```python
from build123d import *

# Parameters (mm, degrees)
SKETCH030_R             = 11
PAD011_DEPTH            = 8.5
SKETCH031_R             = 9.85
PAD012_DEPTH            = 2.5
SKETCH032_R             = 9
POCKET019_DEPTH         = 7.5
SKETCH033_R             = 1.95
POCKET020_DEPTH         = 1.5
FILLET010_R             = 1.2
SKETCH034_R             = 1.1
POCKET021_DEPTH         = 2
SKETCH035_R             = 3.3
POCKET022_DEPTH         = 3.5
SKETCH036_R             = 4.1
POCKET023_DEPTH         = 1.4
BODY011_PLACEMENT_ANGLE = 180.00001


with BuildPart() as part:
    # Sketch030 → Pad011 (new body)
    with BuildSketch(Plane.XY):
        Circle(SKETCH030_R)
    extrude(amount=PAD011_DEPTH)

    # Sketch031 (on Face3 of Pad011) → Pad012 (join)
    with BuildSketch(Plane.XY.offset(8.5)):
        Circle(SKETCH031_R)
    extrude(amount=PAD012_DEPTH)

    # Sketch032 (on Face5 of Pad012) → Pocket019 (cut)
    with BuildSketch(Plane.XY.offset(11)):
        Circle(SKETCH032_R)
    extrude(amount=-POCKET019_DEPTH, mode=Mode.SUBTRACT)

    # Sketch033 (on Face2 of Pocket019) → Pocket020 (cut)
    with BuildSketch(Plane(origin=(0, 0, 0), x_dir=(1, 0, 0), z_dir=(0, 0, -1))):
        with Locations((0, 6.8)):
            Circle(SKETCH033_R)
        with Locations((-5.8889727457, -3.4)):
            Circle(SKETCH033_R)
        with Locations((5.8889727457, -3.4)):
            Circle(SKETCH033_R)
    extrude(amount=-POCKET020_DEPTH, mode=Mode.SUBTRACT)

    # Fillet010
    fillet010_edges = [part.edges().sort_by_distance(p)[0] for p in [
        (-11, 0, 0),
    ]]
    fillet(fillet010_edges, radius=FILLET010_R)

    # Sketch034 (on Face11 of Fillet010) → Pocket021 (cut)
    with BuildSketch(Plane(origin=(0, 0, 1.5), x_dir=(1, 0, 0), z_dir=(0, 0, -1))):
        with Locations((-5.8889727457, -3.4)):
            Circle(SKETCH034_R)
        with Locations((0, 6.8)):
            Circle(SKETCH034_R)
        with Locations((5.8889727457, -3.4)):
            Circle(SKETCH034_R)
    extrude(amount=-POCKET021_DEPTH, mode=Mode.SUBTRACT)

    # Sketch035 (on Face4 of Pocket021) → Pocket022 (cut)
    with BuildSketch(Plane(origin=(0, 0, 0), x_dir=(1, 0, 0), z_dir=(0, 0, -1))):
        Circle(SKETCH035_R)
        with BuildLine():
            ThreePointArc((-3.5353318533, 4.2132444372), (-3.3874236532, 5.9038429005), (-5.0780221165, 6.0517511006))
            ThreePointArc((-5.0780221165, 6.0517511006), (-6.8416006899, 3.95), (-7.7799812488, 1.3718206036))
            ThreePointArc((-7.7799812488, 1.3718206036), (-6.8065897584, -0.0183265132), (-5.4164426416, 0.9550649772))
            ThreePointArc((-3.5353318533, 4.2132444372), (-4.7631397208, 2.75), (-5.4164426416, 0.9550649772))
        make_face()
        with BuildLine():
            ThreePointArc((5.0780221165, 6.0517511006), (3.3874236532, 5.9038429005), (3.5353318533, 4.2132444372))
            ThreePointArc((5.4164426416, 0.9550649772), (4.7631397208, 2.75), (3.5353318533, 4.2132444372))
            ThreePointArc((5.4164426416, 0.9550649772), (6.8065897584, -0.0183265132), (7.7799812488, 1.3718206036))
            ThreePointArc((7.7799812488, 1.3718206036), (6.8416006899, 3.95), (5.0780221165, 6.0517511006))
        make_face()
        with BuildLine():
            ThreePointArc((-1.8811107883, -5.1683094143), (-3.4191661052, -5.8855163873), (-2.7019591323, -7.4235717042))
            ThreePointArc((-2.7019591323, -7.4235717042), (0, -7.9), (2.7019591323, -7.4235717042))
            ThreePointArc((2.7019591323, -7.4235717042), (3.4191661052, -5.8855163873), (1.8811107883, -5.1683094143))
            ThreePointArc((-1.8811107883, -5.1683094143), (0, -5.5), (1.8811107883, -5.1683094143))
        make_face()
    extrude(amount=-POCKET022_DEPTH, mode=Mode.SUBTRACT)

    # Sketch036 (on Face23 of Pocket022) → Pocket023 (cut)
    with BuildSketch(Plane.XY.offset(3.5)):
        Circle(SKETCH036_R)
    extrude(amount=-POCKET023_DEPTH, mode=Mode.SUBTRACT)


with BuildPart() as part_1:
    # Body011 placement: moved
    add(part.part.moved(Location((2.3918e-06, 1e-05, 139.00003))).rotate(Axis((2.3918e-06, 1e-05, 139.00003), (0, 1, 0)), BODY011_PLACEMENT_ANGLE))


solid = part_1.part
```
Part model, mm, in its own coordinate system. A direction names the side the tool comes from. Round coordinates to 2 decimals unless told otherwise and drop trailing zeros.
Item 1: Cut at A-A, the plane x = 0. Count the separate pieces of the cut face and the enclosed holes in it, plus the area to 3 significant figures.
Results:
separate pieces: 4
enclosed holes: 0
area: 56.6 mm2
Item 2: Which spindle directions (+Z, -Z, +X, -X, +Y, -Y) get a long thin tool onto all of the face, cutting with end or side? Do faces 1 (the flat face through (-1, -6, 137.5)), 2 (the flat face through (-3, -9, 128)), 3 (the cylindrical face through (0, 7.9, 137.3)), 4 (the flat face through (-4, 2, 135.5)). Say none if no direction does.
Results:
face 1: +Z
face 2: -Z, +X, -X, +Y, -Y
face 3: +Z, -Z
face 4: -Z
Item 3: Two-plate mould, pull along X, no slides. Class faces 5 (the flat face through (-4, 0, 139)), 6 (the cylindrical face through (6.822, -3.983, 137.275)), 7 (the cylindrical face through (-8.584, 2.703, 131.698)), 8 (the cylindrical face through (2.38, -10.74, 134.2)): +X half, -X half, draft (parallel to the pull), parting line (faces both ways), or undercut.
Results:
face 5: draft
face 6: undercut
face 7: undercut
face 8: parting line
Item 4: Probe L1, parallel to X at y = -1, z = 138; L2, parallel to X at y = 0.25, z = 133.25; L3, parallel to Y at x = -3, z = 137. List the from-to ranges inside material, lowest first.
Results:
L1: x = -10.94 to -7.79, -5.41 to -3.14, 3.14 to 5.41, 7.79 to 10.94
L2: x = -11 to -9, 9 to 11
L3: y = -10.58 to -1.37, 1.37 to 5.33, 7.26 to 10.58
Item 5: Drop flat-ended pins along their axis: pin 1 Ø6 at (y, z) = (8, 131.5) entering from -X; pin 2 Ø5 at (x, y) = (0, -6.8) entering from -Z; pin 3 Ø2.5 at (x, y) = (5.89, 3.4) entering from +Z; pin 4 Ø3 at (x, y) = (-5.89, 3.4) entering from -Z. Give the stop position or say it passes through.
Results:
pin 1: stops at x = -9.8
pin 2: stops at z = 128
pin 3: stops at z = 137.5
pin 4: stops at z = 135.5
